Check sheet for the modelled part. Datum: model origin and axes. Units: mm. Face numbers are marked on the shaded views. A direction names the side the tool comes from. Give positions to 0.01 mm unless a question says otherwise; leave off trailing zeros. Loops run counter-clockwise (first coordinate to the right, second up) from the corner with the lowest first, then second, coordinate; pieces in that order, holes last. Notation, with made-up numbers: (71.5, 50.5) - (105.5, 50.5) arc R8 ccw to (105.5, 59.5) - close; hole circle Ø7 at (-4, 19.25). An arc over 180 degrees is marked (long way). Use one line per item in the form item = value.
from build123d import *

# Parameters (mm, degrees)
SKETCH1_W           = 40
SKETCH1_H           = 40
BOSS_EXTRUDE1_DEPTH = 6
SKETCH2_W           = 12
SKETCH2_H           = 12
CUT_EXTRUDE1_DEPTH  = 2.5
SKETCH3_W           = 12
SKETCH3_H           = 12
CUT_EXTRUDE2_DEPTH  = 2.5
CHAMFER1_SIZE       = 2.5
SKETCH4_W           = 12
SKETCH4_H           = 12
BOSS_EXTRUDE2_DEPTH = 2.5
SKETCH5_W           = 12
SKETCH5_H           = 12
BOSS_EXTRUDE3_DEPTH = 2.5
CHAMFER2_SIZE       = 2.5
SKETCH6_R           = 2.5
CUT_EXTRUDE3_DEPTH  = 2.5
SKETCH7_R           = 1
CUT_EXTRUDE4_DEPTH  = 29.91366459


# Some blends are built 0.0001 mm under size
with BuildPart() as part:
    # Sketch1 → Boss-Extrude1 (new body)
    with BuildSketch(Plane(origin=(0, 0, 0), x_dir=(1, 0, 0), z_dir=(0, 1, 0))):
        Rectangle(SKETCH1_W, SKETCH1_H)
    extrude(amount=BOSS_EXTRUDE1_DEPTH)

    # Sketch2 → Cut-Extrude1 (cut)
    with BuildSketch(Plane.XZ):
        with Locations((14, 14)):
            Rectangle(SKETCH2_W, SKETCH2_H)
        with Locations((-14, 14)):
            Rectangle(SKETCH2_W, SKETCH2_H)
        with Locations((14, -14)):
            Rectangle(SKETCH2_W, SKETCH2_H)
        with Locations((-14, -14)):
            Rectangle(SKETCH2_W, SKETCH2_H)
    extrude(amount=-CUT_EXTRUDE1_DEPTH, mode=Mode.SUBTRACT)

    # Sketch3 → Cut-Extrude2 (cut)
    with BuildSketch(Plane(origin=(0, 6, 0), x_dir=(1, 0, 0), z_dir=(0, 1, 0))):
        with Locations((14, 14)):
            Rectangle(SKETCH3_W, SKETCH3_H)
        with Locations((-14, 14)):
            Rectangle(SKETCH3_W, SKETCH3_H)
        with Locations((14, -14)):
            Rectangle(SKETCH3_W, SKETCH3_H)
        with Locations((-14, -14)):
            Rectangle(SKETCH3_W, SKETCH3_H)
    extrude(amount=-CUT_EXTRUDE2_DEPTH, mode=Mode.SUBTRACT)

    # Chamfer1
    chamfer1_edges = [part.edges().sort_by_distance(p)[0] for p in [
        (-14, 6, -8),
        (-8, 6, -14),
        (0, 6, -20),
        (8, 6, -14),
        (14, 6, -8),
        (20, 6, 0),
        (14, 6, 8),
        (8, 6, 14),
        (0, 6, 20),
        (-8, 6, 14),
        (-14, 6, 8),
        (-20, 6, 0),
        (-20, 0, 0),
        (-14, 0, 8),
        (-8, 0, 14),
        (0, 0, 20),
        (8, 0, 14),
        (14, 0, 8),
        (20, 0, 0),
        (14, 0, -8),
        (8, 0, -14),
        (0, 0, -20),
        (-8, 0, -14),
        (-14, 0, -8),
    ]]
    chamfer(chamfer1_edges, length=CHAMFER1_SIZE - 0.0001)  # a hair under: the kernel refuses the full size

    # Sketch4 → Boss-Extrude2 (add)
    with BuildSketch(Plane.XZ.offset(-2.5)):
        with Locations((14, -14)):
            Rectangle(SKETCH4_W, SKETCH4_H)
        with Locations((14, 14)):
            Rectangle(SKETCH4_W, SKETCH4_H)
        with Locations((-14, -14)):
            Rectangle(SKETCH4_W, SKETCH4_H)
        with Locations((-14, 14)):
            Rectangle(SKETCH4_W, SKETCH4_H)
    extrude(amount=BOSS_EXTRUDE2_DEPTH)

    # Sketch5 → Boss-Extrude3 (add)
    with BuildSketch(Plane(origin=(0, 3.5, 0), x_dir=(1, 0, 0), z_dir=(0, 1, 0))):
        with Locations((-14, -14)):
            Rectangle(SKETCH5_W, SKETCH5_H)
        with Locations((14, -14)):
            Rectangle(SKETCH5_W, SKETCH5_H)
        with Locations((-14, 14)):
            Rectangle(SKETCH5_W, SKETCH5_H)
        with Locations((14, 14)):
            Rectangle(SKETCH5_W, SKETCH5_H)
    extrude(amount=BOSS_EXTRUDE3_DEPTH)

    # Chamfer2
    # the kernel refuses this chamfer: 2.5 mm, written as the material it takes off along each edge
    with BuildSketch(Plane(origin=(8, 6, 8), x_dir=(0, -0.9996219169112968, -0.027495876610586317), z_dir=(1, 0, 0)), Plane(origin=(-26.42920747, 0, -8), x_dir=(0, 0.9996219169112968, 0.027495876610586317), z_dir=(1, 0, 0)), Plane(origin=(-8, 0, 8), x_dir=(0, 0.9996219169112968, -0.027495876610586317), z_dir=(-1, 0, 0)), Plane(origin=(-26.42920747, 6, -8), x_dir=(6.9547671466025935e-15, 0.027495876610586317, -0.9996219169112968), z_dir=(1, 0, 0))) as chamfer2_piece_1:
        Polygon((CHAMFER2_SIZE * 0.999621916911, -CHAMFER2_SIZE * 0.0274958766106), (-CHAMFER2_SIZE * 0.0274958766106, -CHAMFER2_SIZE * 0.999621916911), (0, 0), align=None)
    extrude(amount=18.42920747, mode=Mode.SUBTRACT)
    with BuildSketch(Plane(origin=(20, 6, 1.57079253), x_dir=(0.027495876610586317, -0.9996219169112968, -1.2780451150309794e-15), z_dir=(0, 0, 1)), Plane(origin=(26.42920747, 6, 20), x_dir=(0, -0.9996219169112968, 0.027495876610586317), z_dir=(-1, 0, 0)), Plane(origin=(-20, 0, 1.57079253), x_dir=(-0.027495876610586317, 0.9996219169112968, 0), z_dir=(0, 0, 1)), Plane(origin=(-26.42920747, 0, 20), x_dir=(0, 0.9996219169112968, 0.027495876610586317), z_dir=(1, 0, 0)), Plane(origin=(20, 0, 1.57079253), x_dir=(-0.9996219169112968, -0.027495876610586372, 0), z_dir=(0, 0, 1)), Plane(origin=(26.42920747, 0, -20), x_dir=(0, 0.9996219169112968, -0.027495876610586317), z_dir=(-1, 0, 0)), Plane(origin=(20, 6, -1.57079253), x_dir=(-0.9996219169112968, 0.027495876610586317, -1.0358163835365089e-14), z_dir=(0, 0, -1)), Plane(origin=(-20, 6, -26.42920747), x_dir=(0.9996219169112968, 0.027495876610586317, -3.936102257438915e-14), z_dir=(0, 0, 1)), Plane(origin=(-20, 6, 1.57079253), x_dir=(0.9996219169112968, 0.027495876610586317, 3.5513704578394593e-15), z_dir=(0, 0, 1))) as chamfer2_piece_2:
        Polygon((CHAMFER2_SIZE * 0.999621916911, -CHAMFER2_SIZE * 0.0274958766106), (-CHAMFER2_SIZE * 0.0274958766106, -CHAMFER2_SIZE * 0.999621916911), (0, 0), align=None)
    extrude(amount=24.85841494, mode=Mode.SUBTRACT)
    with BuildSketch(Plane(origin=(8, 6, 26.42920747), x_dir=(0.9996219169112968, 0.027495876610586317, 0), z_dir=(0, 0, -1)), Plane(origin=(-8, 0, -8), x_dir=(-0.9996219169112968, -0.02749587661058636, 0), z_dir=(0, 0, -1)), Plane(origin=(-8, 0, 26.42920747), x_dir=(-0.9996219169112968, -0.027495876610586372, 0), z_dir=(0, 0, -1)), Plane(origin=(8, 0, 26.42920747), x_dir=(-0.027495876610586317, 0.9996219169112968, 0), z_dir=(0, 0, -1)), Plane(origin=(8, 0, -8), x_dir=(0, -0.027495876610586372, -0.9996219169112968), z_dir=(1, 0, 0)), Plane(origin=(8, 0, -26.42920747), x_dir=(0.9996219169112968, -0.027495876610586372, 0), z_dir=(0, 0, 1)), Plane(origin=(8, 6, -8), x_dir=(0, -0.9996219169112968, 0.027495876610586317), z_dir=(1, 0, 0)), Plane(origin=(8, 6, -26.42920747), x_dir=(-0.027495876610586317, -0.9996219169112968, 0), z_dir=(0, 0, 1)), Plane(origin=(-8, 6, 8), x_dir=(0, -0.9996219169112968, -0.027495876610586317), z_dir=(-1, 0, 0)), Plane(origin=(-8, 6, 26.42920747), x_dir=(0.027495876610586317, -0.9996219169112968, 0), z_dir=(0, 0, -1))) as chamfer2_piece_3:
        Polygon((CHAMFER2_SIZE * 0.999621916911, CHAMFER2_SIZE * 0.0274958766106), (-CHAMFER2_SIZE * 0.0274958766106, CHAMFER2_SIZE * 0.999621916911), (0, 0), align=None)
    extrude(amount=18.42920747, mode=Mode.SUBTRACT)
    with BuildSketch(Plane(origin=(-1.57079253, 0, -20), x_dir=(0, -0.027495876610586372, 0.9996219169112968), z_dir=(-1, 0, 0)), Plane(origin=(-20, 0, -26.42920747), x_dir=(0.9996219169112968, -0.027495876610586372, -6.510845839372511e-15), z_dir=(0, 0, 1)), Plane(origin=(26.42920747, 0, 20), x_dir=(0, 0.9996219169112968, 0.027495876610586317), z_dir=(-1, 0, 0)), Plane(origin=(20, 0, -1.57079253), x_dir=(-0.9996219169112968, -0.027495876610586372, 0), z_dir=(0, 0, -1)), Plane(origin=(26.42920747, 6, -20), x_dir=(0, -0.9996219169112968, -0.027495876610586317), z_dir=(-1, 0, 0)), Plane(origin=(-1.57079253, 6, -20), x_dir=(0, -0.9996219169112968, -0.027495876610586317), z_dir=(-1, 0, 0)), Plane(origin=(-26.42920747, 6, 20), x_dir=(1.1722197233405161e-15, -0.9996219169112968, 0.027495876610586317), z_dir=(1, 0, 0))) as chamfer2_piece_4:
        Polygon((CHAMFER2_SIZE * 0.999621916911, CHAMFER2_SIZE * 0.0274958766106), (-CHAMFER2_SIZE * 0.0274958766106, CHAMFER2_SIZE * 0.999621916911), (0, 0), align=None)
    extrude(amount=24.85841494, mode=Mode.SUBTRACT)
    with BuildSketch(Plane(origin=(1.57079253, 0, 8), x_dir=(0, 0.9996219169112968, -0.027495876610586317), z_dir=(1, 0, 0))) as chamfer2_piece_5_section:
        Polygon((CHAMFER2_SIZE * 0.999621916911, CHAMFER2_SIZE * 0.0274958766106), (-CHAMFER2_SIZE * 0.0274958766106, CHAMFER2_SIZE * 0.999621916911), (0, 0), align=None)
    chamfer2_piece_5 = extrude(amount=24.85841494, mode=Mode.PRIVATE)
    chamfer2_piece_5 = split(chamfer2_piece_5, bisect_by=Plane(origin=(9.775276368, 4.275176368, 8.816532421), z_dir=(0.7071067811865475, -0.7071067811865476, -2.3845673236902997e-15)), keep=Keep.TOP, mode=Mode.PRIVATE)
    add(chamfer2_piece_5, mode=Mode.SUBTRACT)
    with BuildSketch(Plane(origin=(-8, 6, -1.57079253), x_dir=(-0.9996219169112968, 0.027495876610586317, -7.028754031140922e-15), z_dir=(0, 0, -1))) as chamfer2_piece_6_section:
        Polygon((CHAMFER2_SIZE * 0.999621916911, -CHAMFER2_SIZE * 0.0274958766106), (-CHAMFER2_SIZE * 0.0274958766106, -CHAMFER2_SIZE * 0.999621916911), (0, 0), align=None)
    chamfer2_piece_6 = extrude(amount=24.85841494, mode=Mode.PRIVATE)
    chamfer2_piece_6 = split(chamfer2_piece_6, bisect_by=Plane(origin=(-8.816532421, 1.724823632, -9.775276368), z_dir=(0, 0.7071067811865476, -0.7071067811865475)), keep=Keep.TOP, mode=Mode.PRIVATE)
    add(chamfer2_piece_6, mode=Mode.SUBTRACT)

    # Sketch6 → Cut-Extrude3 (cut)
    with BuildSketch(Plane.XZ):
        with Locations(Location((14, 14, 0), (0, 0, 270))):
            Circle(SKETCH6_R)
        with Locations(Location((14, -14, 0), (0, 0, 270))):
            Circle(SKETCH6_R)
        with Locations(Location((-14, -14, 0), (0, 0, 270))):
            Circle(SKETCH6_R)
        with Locations(Location((-14, 14, 0), (0, 0, 270))):
            Circle(SKETCH6_R)
    extrude(amount=-CUT_EXTRUDE3_DEPTH, mode=Mode.SUBTRACT)

    # Sketch7 → Cut-Extrude4 (cut, through all)
    with BuildSketch(Plane(origin=(0, 6, 0), x_dir=(1, 0, 0), z_dir=(0, 1, 0))):
        with Locations(Location((0, 0, 0), (0, 0, 270))):
            Circle(SKETCH7_R)
    extrude(amount=-CUT_EXTRUDE4_DEPTH, mode=Mode.SUBTRACT)


solid = part.part
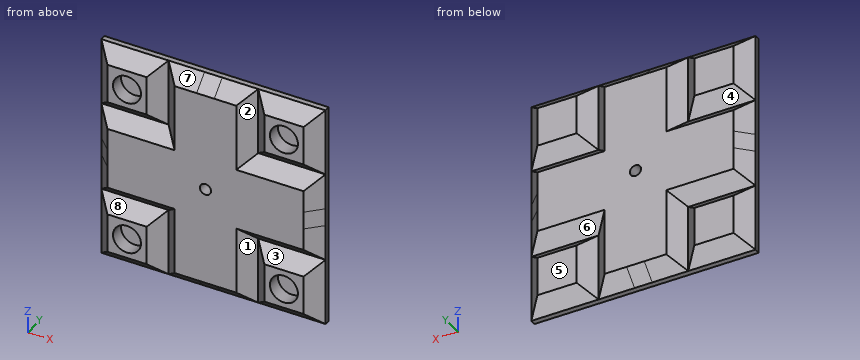
Item 1: Access from +Z, -Z, +X, -X, +Y, -Y to the whole of each face (thin tool, end or side, straight path). Record for the marked faces 1, 2, 3 and 4.
Answer block:
face_1 = -Z, -Y
face_2 = +Z, -Y
face_3 = +X, -Y
face_4 = -X, +Y
Item 2: Thickness scan on L1, parallel to X at y = 0.5, z = -11; L2, parallel to X at y = 0.9, z = -14; L3, parallel to Z at x = 15, y = 4. Record the ranges inside material, lowest first.
Answer block:
L1 = -18 to -10, -6 to 6, 10 to 18
L2 = -18.4 to -16.5, -11.5 to -9.6, -6.4 to 6.4, 9.6 to 11.5, 16.5 to 18.4
L3 = -19.5 to -8.5, -7.5 to 7.5, 8.5 to 19.5
Item 3: Section check D-D on x = -9. Record the boundary of the cut face in (y, z).
Answer block:
outline = (0, -5.5) - (2.5, -8) - (1.5, -9) - (1.5, -19) - (2.5, -20) - (3.5, -20) - (4.5, -19) - (4.5, -9) - (3.5, -8) - (6, -5.5) - (6, 5.5) - (3.5, 8) - (4.5, 9) - (4.5, 19) - (3.5, 20) - (2.5, 20) - (1.5, 19) - (1.5, 9) - (2.5, 8) - (0, 5.5) - close
Item 4: Gauge pin test, flat ends, axial feed: P1, Ø3, axis at x = 14, z = 14, coming from the -Y side; P2, Ø2, axis at x = 7, z = 12.5, coming from the -Y side; P3, Ø0.7, axis at y = 1.5, z = -18.5, coming from the -X side. Record the tip position at first contact, or that the pin passes through.
Answer block:
P1 = 2.5
P2 = 0.5
P3 = -19.35
Item 5: Section check A-A on z = 0. Record the boundary of the cut face in (x, y).
Answer block:
outline = (-20, 2.5) - (-17.5, 0) - (-1, 0) - (-1, 6) - (-17.5, 6) - (-20, 3.5) - close; (1, 0) - (17.5, 0) - (20, 2.5) - (20, 3.5) - (17.5, 6) - (1, 6) - close
Item 6: Mould release check, pull along Z, two halves, no side actions. Record for the marked faces 5, 6, 7 and 8: released by +Z, released by -Z, zero draft, split by the parting line, or undercut.
Answer block:
face_5 = zero draft
face_6 = undercut
face_7 = released by +Z
face_8 = undercut
Item 7: Section check B-B on x = 0. Record the boundary of the cut face in (y, z), then the cut area to 3 significant figures.
Answer block:
outline = (0, -17.5) - (2.5, -20) - (3.5, -20) - (6, -17.5) - (6, -1) - (0, -1) - close; (0, 1) - (6, 1) - (6, 17.5) - (3.5, 20) - (2.5, 20) - (0, 17.5) - close
area = 216 mm2
Item 8: Section check C-C on y = 1.5. Give the number of separate pieces and of enclosed holes in the cut face, then the cut area to 3 significant figures.
Answer block:
separate_pieces = 5
enclosed_holes = 5
area = 1,190 mm2
